from build123d import *

# Parameters (mm, degrees)
SKETCH1_R               = 4.85
BOSS_EXTRUDE1_DEPTH     = 103.5535633
CUT_EXTRUDE1_DEPTH      = 104.780467681
CUT_EXTRUDE1_DEPTH_BACK = 104.780467681
SKETCH2_R               = 1.25
CUT_EXTRUDE2_DEPTH      = 104.78046779
CUT_EXTRUDE2_DEPTH_BACK = 104.78046779
SKETCH3_W               = 42.028968594
SKETCH3_H               = 71.494930271
SCALE1_SCALE            = 1.5


with BuildPart() as part:
    # Sketch1 → Boss-Extrude1 (new body)
    with BuildSketch(Plane(origin=(0, 0, 0), x_dir=(0, 0, -1), z_dir=(1, 0, 0))):
        Circle(SKETCH1_R)
    extrude(amount=BOSS_EXTRUDE1_DEPTH)

    # Sketch2 → Cut-Extrude1 (cut, two sides: drawn at the far end of the back side and taken through both)
    with BuildSketch(Plane.XY.offset(-CUT_EXTRUDE1_DEPTH_BACK)):
        with Locations((101.0535633, 0)):
            Circle(SKETCH2_R)
    extrude(amount=CUT_EXTRUDE1_DEPTH + CUT_EXTRUDE1_DEPTH_BACK, mode=Mode.SUBTRACT)

    # Sketch3 → Cut-Extrude2 (cut, two sides: drawn at the far end of the back side and taken through both)
    with BuildSketch(Plane(origin=(0, 0, 0), x_dir=(1, 0, 0), z_dir=(0, 1, 0)).offset(-CUT_EXTRUDE2_DEPTH_BACK)):
        with Locations((-11.495089548, 16.503222723)):
            Rectangle(SKETCH3_W, SKETCH3_H)
    extrude(amount=CUT_EXTRUDE2_DEPTH + CUT_EXTRUDE2_DEPTH_BACK, mode=Mode.SUBTRACT)


with BuildPart() as part_1:
    # Scale1: scaled about (56.231945049, 6e-09, 2.83e-07)
    add(part.part.scale(SCALE1_SCALE).moved(Location((-28.115972524, -3e-09, -1.41e-07))))


solid = part_1.part
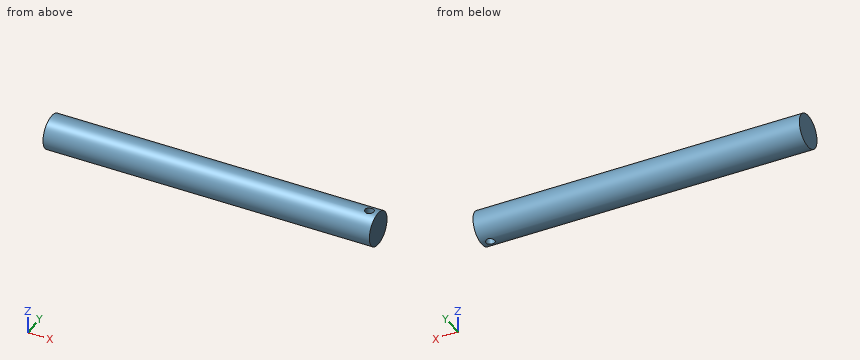
Read the model definition and answer for the solid it produces. Units are mm, in the model's axes. Round coordinates to 2 decimals unless told otherwise and drop trailing zeros. Write each loop counter-clockwise with the first axis right and the second up, starting at its lowest first coordinate (ties: lowest second). Pieces come first, ordered by that corner, then holes. Notation, with made-up numbers: M 24,18 L 42,18 A25 cw 42,45 Z; hole C 13.25,29.25 d4. An arc over 180 degrees is marked long. Use a Markdown table: item, result.
1) The part is cut by section D-D (y = 5.5). Write down the section's boundary in (x, z).
Answers follow:
| item | result |
|---|---|
| outline | M -13.84,-4.76 L 127.21,-4.76 L 127.21,4.76 L -13.84,4.76 Z |
2) Straight lines are drawn through the part: line 1 along X through (y, z) = (0, -2); line 2 along X through (y, z) = (0.5, 3.5); line 3 along Y through (x, z) = (33, -5.25). For each, find the intervals that lie inside material, in ascending order. Write a range as [from, to].
Answers follow:
| item | result |
|---|---|
| line 1 | x = [-13.84, 121.59], [125.34, 127.21] |
| line 2 | x = [-13.84, 121.66], [125.27, 127.21] |
| line 3 | y = [-5.04, 5.04] |
3) Flat-ended cylindrical pins translate along their axes: pin 1 (6 mm diameter, centred on x = 11.5, z = -3.5, fed in from +Y); pin 2 (2 mm diameter, centred on x = 70, z = -5, fed in from -Y); pin 3 (2 mm diameter, centred on x = 63.5, y = -3.5, fed in from +Z). Find the tip coordinate at first contact, or state that the pin passes through.
Answers follow:
| item | result |
|---|---|
| pin 1 | stops at y = 7.26 |
| pin 2 | stops at y = -6.08 |
| pin 3 | stops at z = 6.83 |
4) The part is cut by section B-B (z = -1.5). Write down the section's boundary in (x, y) (3 decimals).
Answers follow:
| item | result |
|---|---|
| outline | M -13.837,-7.119 L 127.214,-7.119 L 127.214,7.119 L -13.837,7.119 Z; hole C 123.464,0 d3.75 |
5) The part is cut by section C-C (x = -3). Write down the section's boundary in (y, z) (3 decimals).
Answers follow:
| item | result |
|---|---|
| outline | C 0,0 d14.55 |
6) The part is cut by section A-A (y = 0). Write down the section's boundary in (x, z) (3 decimals), plus the area to 3 significant figures.
Answers follow:
| item | result |
|---|---|
| outline | M -13.837,-7.275 L 121.589,-7.275 L 121.589,7.275 L -13.837,7.275 Z; M 125.339,-7.275 L 127.214,-7.275 L 127.214,7.275 L 125.339,7.275 Z |
| area | 2,000 mm2 |
